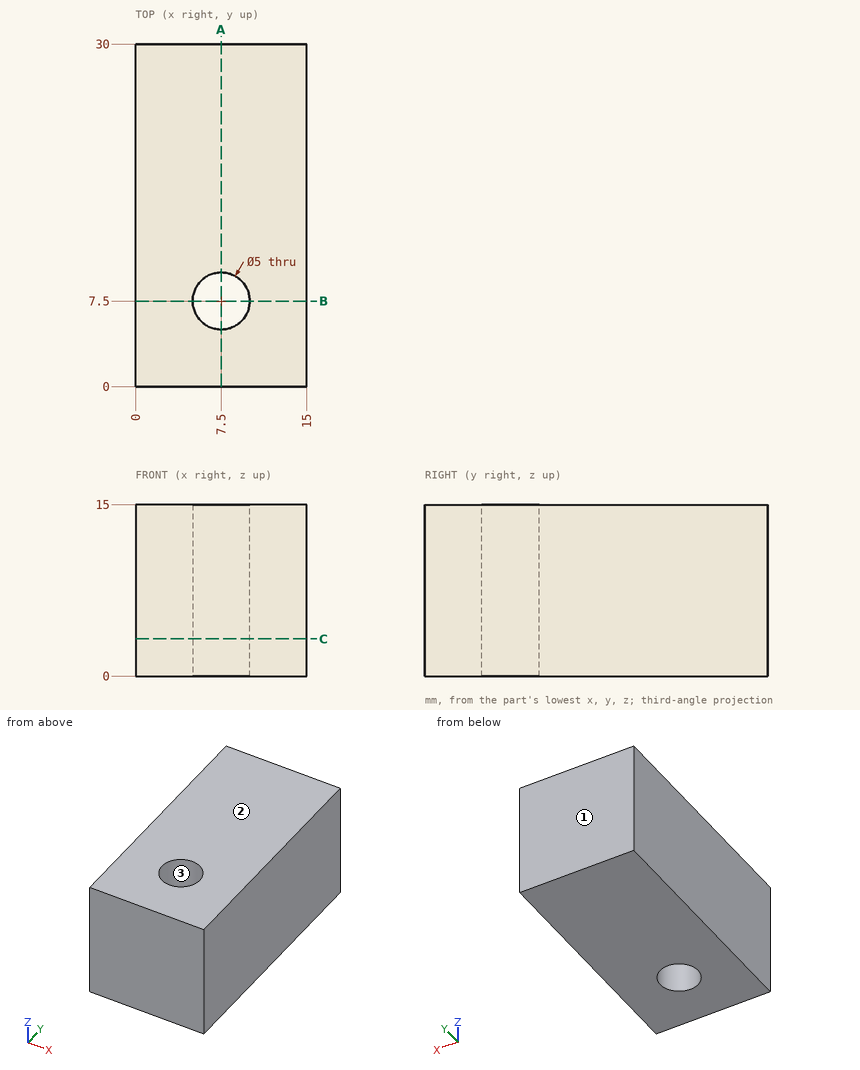
Print and shaded views of the part. All mm, measured from the part's lowest x, y and z. Coordinates: 2 decimals unless noted, no trailing zeros. Loops run counter-clockwise (first coordinate to the right, second up) from the corner with the lowest first, then second, coordinate; pieces in that order, holes last. Notation, with made-up numbers: (27, 16) - (66, 16) arc R12 ccw to (66, 29) - close; hole circle Ø4 at (-14, 19). An arc over 180 degrees is marked (long way). Write item = value, one per line. Start each with the question number.
Item 1: Mould opens along Y. For the marked faces 1, 2 and 3 say: released by +Y, released by -Y, zero draft, split by the parting line, or undercut.
Item 2: Wall check: L1, parallel to X at y = 7.5, z = 4.75; L2, parallel to Y at x = 7.5, z = 7.5; L3, parallel to X at y = 5.75, z = 14. Give the ranges that are in metal, low to high. Write a range as from..to.
Item 3: Cut at C-C, the plane z = 3.25. Give the cut face in (x, y), and give its area (3 significant figures).
Item 4: Cut at A-A, the plane x = 7.5. Give the cut face in (y, z), and give its area (3 significant figures).
Item 5: Cut at B-B, the plane y = 7.5. Give the cut face in (x, z), and give its area (3 significant figures).
The answers:
q1.face_1 = released by +Y
q1.face_2 = zero draft
q1.face_3 = undercut
q2.L1 = 0..5, 10..15
q2.L2 = 0..5, 10..30
q2.L3 = 0..5.71, 9.29..15
q3.outline = (0, 0) - (15, 0) - (15, 30) - (0, 30) - close; hole circle Ø5 at (7.5, 7.5)
q3.area = 430 mm2
q4.outline = (0, 0) - (5, 0) - (5, 15) - (0, 15) - close; (10, 0) - (30, 0) - (30, 15) - (10, 15) - close
q4.area = 375 mm2
q5.outline = (0, 0) - (5, 0) - (5, 15) - (0, 15) - close; (10, 0) - (15, 0) - (15, 15) - (10, 15) - close
q5.area = 150 mm2
